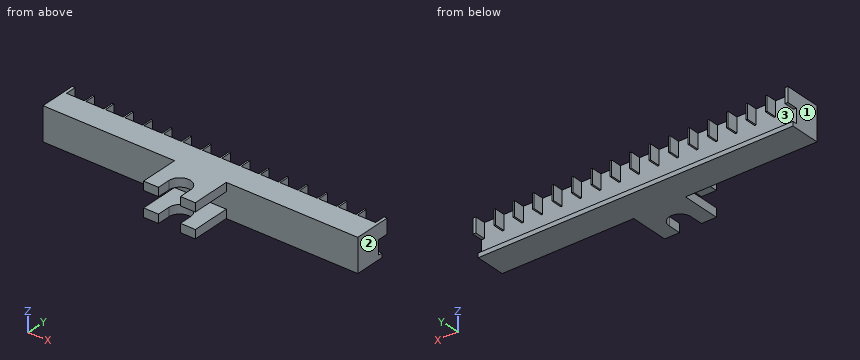
from build123d import *

# Parameters (mm, degrees)
SKETCH1_W                       = 73
SKETCH1_H                       = 7.715
BOSS_EXTRUDE1_DEPTH             = 6
SKETCH2_W                       = 73
SKETCH2_H                       = 1
BOSS_EXTRUDE2_DEPTH             = 1
SKETCH3_W                       = 0.35
SKETCH3_H                       = 7.715
BOSS_EXTRUDE3_DEPTH             = 2.5
BOSS_EXTRUDE4_REACH             = 40.165
SKETCH4_W                       = 0.325
SKETCH4_H                       = 2.5
BOSS_EXTRUDE4_DIRECTION_2_REACH = 40.165
BOSS_EXTRUDE5_REACH             = 40.165
BOSS_EXTRUDE5_DIRECTION_2_REACH = 40.165
SKETCH6_W                       = 12
SKETCH6_H                       = 3.715
CUT_EXTRUDE1_DEPTH              = 9
CUT_EXTRUDE2_DEPTH              = 39.279318502
CUT_EXTRUDE2_DEPTH_BACK         = 39.279318502


with BuildPart() as part:
    # Sketch1 → Boss-Extrude1 (new body)
    with BuildSketch(Plane(origin=(0, 0, 0), x_dir=(1, 0, 0), z_dir=(0, 1, 0))):
        with Locations((0, -3.3575)):
            Rectangle(SKETCH1_W, SKETCH1_H)
    extrude(amount=BOSS_EXTRUDE1_DEPTH)

    # Sketch2 → Boss-Extrude2 (add)
    with BuildSketch(Plane(origin=(0, 6, 0), x_dir=(1, 0, 0), z_dir=(0, 1, 0))):
        Rectangle(SKETCH2_W, SKETCH2_H)
    extrude(amount=BOSS_EXTRUDE2_DEPTH)

    # Sketch3 → Boss-Extrude3 (add)
    with BuildSketch(Plane(origin=(0, 6, 0), x_dir=(1, 0, 0), z_dir=(0, 1, 0))):
        with Locations((4.5, -3.3575)):
            Rectangle(SKETCH3_W, SKETCH3_H)
        with Locations((0, -3.3575)):
            Rectangle(SKETCH3_W, SKETCH3_H)
        with Locations((9, -3.3575)):
            Rectangle(SKETCH3_W, SKETCH3_H)
        with Locations((13.5, -3.3575)):
            Rectangle(SKETCH3_W, SKETCH3_H)
        with Locations((18, -3.3575)):
            Rectangle(SKETCH3_W, SKETCH3_H)
        with Locations((22.5, -3.3575)):
            Rectangle(SKETCH3_W, SKETCH3_H)
        with Locations((27, -3.3575)):
            Rectangle(SKETCH3_W, SKETCH3_H)
        with Locations((31.5, -3.3575)):
            Rectangle(SKETCH3_W, SKETCH3_H)
        with Locations((36, -3.3575)):
            Rectangle(SKETCH3_W, SKETCH3_H)
        with Locations((-4.5, -3.3575)):
            Rectangle(SKETCH3_W, SKETCH3_H)
        with Locations((-9, -3.3575)):
            Rectangle(SKETCH3_W, SKETCH3_H)
        with Locations((-13.5, -3.3575)):
            Rectangle(SKETCH3_W, SKETCH3_H)
        with Locations((-18, -3.3575)):
            Rectangle(SKETCH3_W, SKETCH3_H)
        with Locations((-22.5, -3.3575)):
            Rectangle(SKETCH3_W, SKETCH3_H)
        with Locations((-27, -3.3575)):
            Rectangle(SKETCH3_W, SKETCH3_H)
        with Locations((-31.5, -3.3575)):
            Rectangle(SKETCH3_W, SKETCH3_H)
        with Locations((-36, -3.3575)):
            Rectangle(SKETCH3_W, SKETCH3_H)
    extrude(amount=BOSS_EXTRUDE3_DEPTH)

    # Boss-Extrude4: up to this face of the body (flat: up to its plane)
    boss_extrude4_end = Plane(part.part.faces().sort_by_distance((0, 3.139594259, 7.215))[0])
    # Sketch4 → Boss-Extrude4 (add, up to the picked face)
    with BuildSketch(Plane.XY, mode=Mode.PRIVATE) as boss_extrude4_sk1:
        with Locations((36.3375, 7.25)):
            Rectangle(SKETCH4_W, SKETCH4_H)
    boss_extrude4_tool1 = split(extrude(boss_extrude4_sk1.sketch, amount=BOSS_EXTRUDE4_REACH, mode=Mode.PRIVATE), bisect_by=boss_extrude4_end, keep=Keep.BOTH, mode=Mode.PRIVATE)
    # Sketch4 → Boss-Extrude4 (add, up to the picked face)
    with BuildSketch(Plane.XY, mode=Mode.PRIVATE) as boss_extrude4_sk2:
        with Locations((-36.3375, 7.25)):
            Rectangle(SKETCH4_W, SKETCH4_H)
    boss_extrude4_tool2 = split(extrude(boss_extrude4_sk2.sketch, amount=BOSS_EXTRUDE4_REACH, mode=Mode.PRIVATE), bisect_by=boss_extrude4_end, keep=Keep.BOTH, mode=Mode.PRIVATE)
    add(boss_extrude4_tool1.solids().sort_by(Axis((36.3375, 7.25, 0), (0, 0, 1)))[0])
    add(boss_extrude4_tool2.solids().sort_by(Axis((-36.3375, 7.25, 0), (0, 0, 1)))[0])

    # Boss-Extrude4 direction 2: up to this face of the body (flat: up to its plane)
    boss_extrude4_direction_2_end = Plane(part.part.faces().sort_by_distance((0, 3.572955234, -0.5))[0])
    # Sketch4 → Boss-Extrude4 direction 2 (add, up to the picked face)
    with BuildSketch(Plane.XY, mode=Mode.PRIVATE) as boss_extrude4_direction_2_sk1:
        with Locations((36.3375, 7.25)):
            Rectangle(SKETCH4_W, SKETCH4_H)
    boss_extrude4_direction_2_tool1 = split(extrude(boss_extrude4_direction_2_sk1.sketch, amount=-BOSS_EXTRUDE4_DIRECTION_2_REACH, mode=Mode.PRIVATE), bisect_by=boss_extrude4_direction_2_end, keep=Keep.BOTH, mode=Mode.PRIVATE)
    # Sketch4 → Boss-Extrude4 direction 2 (add, up to the picked face)
    with BuildSketch(Plane.XY, mode=Mode.PRIVATE) as boss_extrude4_direction_2_sk2:
        with Locations((-36.3375, 7.25)):
            Rectangle(SKETCH4_W, SKETCH4_H)
    boss_extrude4_direction_2_tool2 = split(extrude(boss_extrude4_direction_2_sk2.sketch, amount=-BOSS_EXTRUDE4_DIRECTION_2_REACH, mode=Mode.PRIVATE), bisect_by=boss_extrude4_direction_2_end, keep=Keep.BOTH, mode=Mode.PRIVATE)
    add(boss_extrude4_direction_2_tool1.solids().sort_by(Axis((36.3375, 7.25, 0), (0, 0, -1)))[0])
    add(boss_extrude4_direction_2_tool2.solids().sort_by(Axis((-36.3375, 7.25, 0), (0, 0, -1)))[0])

    # Boss-Extrude5: up to this face of the body (flat: up to its plane)
    boss_extrude5_end = Plane(part.part.faces().sort_by_distance((0, 3.154290429, 7.215))[0])
    # Sketch5 → Boss-Extrude5 (add, up to the picked face)
    with BuildSketch(Plane.XY, mode=Mode.PRIVATE) as boss_extrude5_sk1:
        with BuildLine():
            Line((-2.54, -6), (-2.54, -9))
            Line((-2.54, -9), (-6, -9))
            Line((-6, -9), (-6, 0))
            Line((-6, 0), (6, 0))
            Line((6, 0), (6, -9))
            Line((6, -9), (2.54, -9))
            Line((2.54, -9), (2.54, -6))
            ThreePointArc((2.54, -6), (0, -3.46), (-2.54, -6))
        make_face()
    boss_extrude5_tool1 = split(extrude(boss_extrude5_sk1.sketch, amount=BOSS_EXTRUDE5_REACH, mode=Mode.PRIVATE), bisect_by=boss_extrude5_end, keep=Keep.BOTH, mode=Mode.PRIVATE)
    add(boss_extrude5_tool1.solids().sort_by(Axis((-2.69, -7.5, 0), (0, 0, 1)))[0])

    # Boss-Extrude5 direction 2: up to this face of the body (flat: up to its plane)
    boss_extrude5_direction_2_end = Plane(part.part.faces().sort_by_distance((0, 3.580773661, -0.5))[0])
    # Sketch5 → Boss-Extrude5 direction 2 (add, up to the picked face)
    with BuildSketch(Plane.XY, mode=Mode.PRIVATE) as boss_extrude5_direction_2_sk1:
        with BuildLine():
            Line((-2.54, -6), (-2.54, -9))
            Line((-2.54, -9), (-6, -9))
            Line((-6, -9), (-6, 0))
            Line((-6, 0), (6, 0))
            Line((6, 0), (6, -9))
            Line((6, -9), (2.54, -9))
            Line((2.54, -9), (2.54, -6))
            ThreePointArc((2.54, -6), (0, -3.46), (-2.54, -6))
        make_face()
    boss_extrude5_direction_2_tool1 = split(extrude(boss_extrude5_direction_2_sk1.sketch, amount=-BOSS_EXTRUDE5_DIRECTION_2_REACH, mode=Mode.PRIVATE), bisect_by=boss_extrude5_direction_2_end, keep=Keep.BOTH, mode=Mode.PRIVATE)
    add(boss_extrude5_direction_2_tool1.solids().sort_by(Axis((-2.69, -7.5, 0), (0, 0, -1)))[0])

    # Sketch6 → Cut-Extrude1 (cut)
    with BuildSketch(Plane.XZ.offset(9)):
        with Locations((0, 3.3575)):
            Rectangle(SKETCH6_W, SKETCH6_H)
    extrude(amount=-CUT_EXTRUDE1_DEPTH, mode=Mode.SUBTRACT)

    # Sketch7 → Cut-Extrude2 (cut, two sides: drawn at the far end of the back side and taken through both)
    with BuildSketch(Plane(origin=(0, 0, 0), x_dir=(0, 0, -1), z_dir=(1, 0, 0)).offset(-CUT_EXTRUDE2_DEPTH_BACK)):
        Polygon((0.5, 7), (-0.5, 7), (-0.5, 6), (-3.802, 6), (-3.802, 8.5), (0.5, 8.5), align=None)
    extrude(amount=CUT_EXTRUDE2_DEPTH + CUT_EXTRUDE2_DEPTH_BACK, mode=Mode.SUBTRACT)


solid = part.part
Can you work these out from the model? Positions are in its coordinate system, mm. Face numbers are marked on the shaded views. Give positions to 0.01 mm unless a question says otherwise; leave off trailing zeros. Order: outer loops, then holes, each group sorted by start corner. A loop starts at its lowest first (then second) coordinate and runs counter-clockwise, first axis right, second up. Notation, with made-up numbers: M -34,-32 L -4,-32 A13 ccw -4,-28 Z; hole C -23,5.5 d6. An arc over 180 degrees is marked long. Use one line per item in the form item = value.
Item 1: If we section it at B-B, the plane z = 2.25: Write out the boundary of the cut face in (x, y), and give its area (3 significant figures).
Values follow:
outline = M -36.5,0 L 36.5,0 L 36.5,6 L -36.5,6 Z
area = 438 mm^2
Item 2: If we section it at A-A, the plane x = 16: Write out the boundary of the cut face in (y, z) (3 decimals).
Values follow:
outline = M 0,-0.5 L 7,-0.5 L 7,0.5 L 6,0.5 L 6,7.215 L 0,7.215 Z
Item 3: Will these pins go through, and if not, where does the flat tip stop? pin 1 Ø3 at (x, z) = (26.5, 4) entering from +Y; pin 2 Ø4 at (y, z) = (-5.5, 1) entering from +X; pin 3 Ø0.6 at (y, z) = (-7, 6) entering from -X.
Values follow:
pin_1 = 8.5
pin_2 = 6
pin_3 = -6
Item 4: Thinking about a two-plate mould opening in X: for the marked faces 1, 2 and 3, which applies, pulls with the +X half, pulls with the -X half, needs draft (parallel to the pull), parting line crosses it, or undercut?
Values follow:
face_1 = pulls with the -X half
face_2 = pulls with the +X half
face_3 = undercut
Item 5: If I drill on line 1 along X through (y, z) = (-7.25, 1.25); line 2 along Z through (x, y) = (-4, -4.25) (3 decimals); line 3 along Y through (x, z) = (-20.5, 5.75), over which ranges is the centre line in solid material (lowest first)? Write a range as [from, to].
Values follow:
line_1 = [-6, -2.54], [2.54, 6]
line_2 = [-0.5, 1.5], [5.215, 7.215]
line_3 = [0, 6]
